Read the model definition and answer for the solid it produces. Units are mm, in the model's axes. Face numbers are marked on the shaded views. A direction names the side the tool comes from. Round coordinates to 2 decimals unless told otherwise and drop trailing zeros. Write each loop counter-clockwise with the first axis right and the second up, starting at its lowest first coordinate (ties: lowest second). Pieces come first, ordered by that corner, then holes. Notation, with made-up numbers: (8, -25) -> (12, -25) arc R17 ccw to (12, -6) -> close; hole circle Ø3 at (30, 51). An arc over 180 degrees is marked (long way). Return JSON: item names as keys, results as strings.
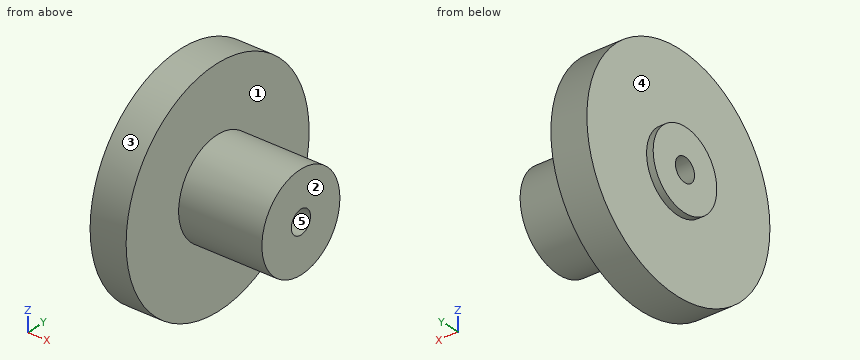
Autodesk Inventor part; units mm, degrees
ref_plane "YZ Plane" through (0, 0, 0) normal (1, 0, 0) x (0, 1, 0)
ref_plane "XZ Plane" through (0, 0, 0) normal (0, 1, 0) x (-1, 0, 0)
ref_plane "XY Plane" through (0, 0, 0) normal (0, 0, 1) x (1, 0, 0)
sketch "Sketch1" plane through (0, 0, 0) normal (0, 0, 1) x (1, 0, 0)
  line L0 (0.34, 5.75) -> (2.2, 5.75)
  line L1 (2.2, 5.75) -> (2.2, 2.45)
  line L2 (2.2, 2.45) -> (6.5, 2.45)
  line L3 (6.5, 2.45) -> (6.5, 0)
  line L4 (6.5, 0) -> (0, 0)
  line L5 (0, 0) -> (0, 2)
  line L6 (0, 2) -> (0.34, 2)
  line L7 (0.34, 2) -> (0.34, 5.75)
  dimension "d2" = 4.9
  dimension "d3" = 11.5
  dimension "d4" = 1.86
  dimension "d5" = 4
  dimension "d6" = 4.3
  dimension "d7" = 6.5
revolve "Revolution1" add sketch "Sketch1" angle 360 about axis through (6.5, 0, 0) along (-1, 0, 0)
hole "Hole1" at (6.5, 0, 0) direction (-1, 0, 0) diameter 1.2 end through all
properties part number "Hitec HS-225MG gear 4"
Item 1: For a pull along Z with two mould halves and no side action, classify the marked faces 3, 4 and 5 as released by +Z, released by -Z, zero draft, split by the parting line, or undercut.
Worked answers:
{"face 3": "split by the parting line", "face 4": "zero draft", "face 5": "undercut"}
Item 2: Section A-A (z = 0) is taken. Give the vertices of the cut face in (x, y), then the cut area to 3 significant figures.
Worked answers:
{"outline": "(0, -2) -> (0.34, -2) -> (0.34, -5.75) -> (2.2, -5.75) -> (2.2, -2.45) -> (6.5, -2.45) -> (6.5, -0.6) -> (0, -0.6) -> close; (0, 0.6) -> (6.5, 0.6) -> (6.5, 2.45) -> (2.2, 2.45) -> (2.2, 5.75) -> (0.34, 5.75) -> (0.34, 2) -> (0, 2) -> close", "area": "36.0 mm2"}
Item 3: Straight lines are drawn through the part: L1, parallel to Y at x = 1.75, z = 0; L2, parallel to Y at x = 2.5, z = 0. For each, find the intervals that lie inside material, in ascending order. Write a range as [from, to].
Worked answers:
{"L1": "y = [-5.75, -0.6], [0.6, 5.75]", "L2": "y = [-2.45, -0.6], [0.6, 2.45]"}
Item 4: A tool of negligible diameter and unlimited length cuts with its end or side. For the marked faces 1 and 2, from which of +Z, -Z, +X, -X, +Y, -Y can it reach the whole face along a straight path? Write none if from no direction.
Worked answers:
{"face 1": "+X", "face 2": "+Z, -Z, +X, +Y, -Y"}
Item 5: Section D-D (z = 1.75) is taken. Give the vertices of the cut face in (x, y).
Worked answers:
{"outline": "(0, -0.97) -> (0.34, -0.97) -> (0.34, -5.48) -> (2.2, -5.48) -> (2.2, -1.71) -> (6.5, -1.71) -> (6.5, 1.71) -> (2.2, 1.71) -> (2.2, 5.48) -> (0.34, 5.48) -> (0.34, 0.97) -> (0, 0.97) -> close"}
Item 6: Section C-C (x = 5.25) is taken. Give the vertices of the cut face in (y, z), then the cut area to 3 significant figures.
Worked answers:
{"outline": "circle Ø4.9 at (0, 0); hole circle Ø1.2 at (0, 0)", "area": "17.7 mm2"}
Item 7: A flat-ended cylindrical pin translates along its axis: pin 1 (1.5 mm diameter, centred on x = 4, y = 4, fed in from -Z). Find the tip coordinate at first contact, or state that the pin passes through.
Worked answers:
{"pin 1": "passes through"}
